Design review of the part built by this model. Coordinates are the model's own, in mm. Face numbers are marked on the shaded views. A direction names the side the tool comes from. Give positions to 0.01 mm unless a question says otherwise; leave off trailing zeros. Loops run counter-clockwise (first coordinate to the right, second up) from the corner with the lowest first, then second, coordinate; pieces in that order, holes last. Notation, with made-up numbers: (86, 47.5) -> (117, 47.5) arc R10 cw to (117, 57.5) -> close; hole circle Ø8 at (19.25, 5.25). An arc over 180 degrees is marked (long way). Answer in a Markdown table with one row per item. Add a question column.
(1) For line 1 (X direction, y = -5, z = 21.25); line 2 (Y direction, x = 7.75, z = 1), list the stretches that pass through material, from the lowest coordinate up.
(2) Consider section B-B on x = 4.5. Write out the cut boundary in (y, z).
(3) For the marked faces 1 and 2, list the 3-axis set-ups (+Z, -Z, +X, -X, +Y, -Y) from which the entire face can be reached by the end or side of a thin tool; tool diameter is ignored.
(4) Consider section D-D on x = 10. Write out the cut boundary in (y, z), then the cut area to 3 significant figures.
(5) Consider section A-A on z = 14. Write out the cut boundary in (x, y), then the cut area to 3 significant figures.
(6) Consider section C-C on z = 23. Write out the cut boundary in (x, y).
(7) For pin 1 (10 mm diameter, centred on x = 23.5, z = 11, fed in from +Y); pin 2 (7.5 mm diameter, centred on y = -48, z = 7, fed in from +X); pin 3 (8 mm diameter, centred on x = 13.5, y = -8.5, fed in from -Z) (1 decimal), all flat-tipped, find the tip position at first contact; note any pin that passes through.
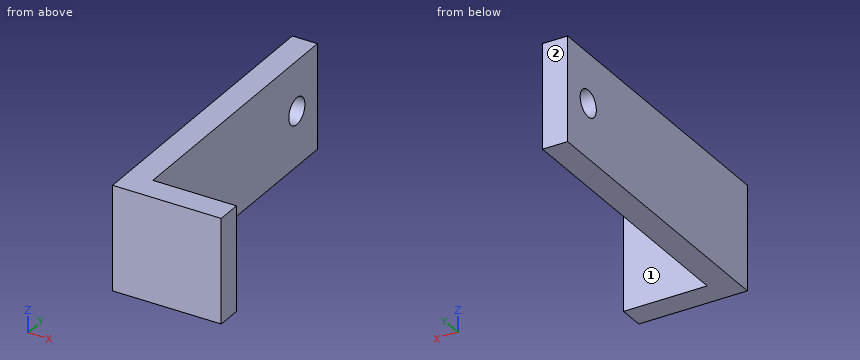
from build123d import *

# Parameters (mm, degrees)
SKETCH1_W           = 25
SKETCH1_H           = 71
BOSS_EXTRUDE1_DEPTH = 6
SKETCH2_W           = 25
SKETCH2_H           = 6
BOSS_EXTRUDE2_DEPTH = 20
SKETCH3_R           = 3.187620356
CUT_EXTRUDE1_DEPTH  = 22.5


with BuildPart() as part:
    # Sketch1 → Boss-Extrude1 (new body)
    with BuildSketch(Plane(origin=(0, 0, 0), x_dir=(0, 0, -1), z_dir=(1, 0, 0))):
        with Locations((-12.5, -35.5)):
            Rectangle(SKETCH1_W, SKETCH1_H)
    extrude(amount=BOSS_EXTRUDE1_DEPTH)

    # Sketch2 → Boss-Extrude2 (add)
    with BuildSketch(Plane(origin=(6, 0, 0), x_dir=(0, 0, -1), z_dir=(1, 0, 0))):
        with Locations((-12.5, -68)):
            Rectangle(SKETCH2_W, SKETCH2_H)
    extrude(amount=BOSS_EXTRUDE2_DEPTH)

    # Sketch3 → Cut-Extrude1 (cut)
    with BuildSketch(Plane(origin=(6, 0, 0), x_dir=(0, 0, -1), z_dir=(1, 0, 0))):
        with Locations((-13.070218864, -8.129494521)):
            Circle(SKETCH3_R)
    extrude(amount=-CUT_EXTRUDE1_DEPTH, mode=Mode.SUBTRACT)


solid = part.part
Values follow:
| question | item | result |
|---|---|---|
| 1 | line 1 | 0 to 6 |
| 1 | line 2 | -71 to -65 |
| 2 | outline | (-71, 0) -> (0, 0) -> (0, 25) -> (-71, 25) -> close; hole circle Ø6.38 at (-8.13, 13.07) |
| 3 | face 1 | +Z, -Z, +X, +Y |
| 3 | face 2 | +Z, -Z, +X, -X, +Y |
| 4 | outline | (-71, 0) -> (-65, 0) -> (-65, 25) -> (-71, 25) -> close |
| 4 | area | 150 mm2 |
| 5 | outline | (0, -71) -> (26, -71) -> (26, -65) -> (6, -65) -> (6, -11.18) -> (0, -11.18) -> close; (0, -5.08) -> (6, -5.08) -> (6, 0) -> (0, 0) -> close |
| 5 | area | 509 mm2 |
| 6 | outline | (0, -71) -> (26, -71) -> (26, -65) -> (6, -65) -> (6, 0) -> (0, 0) -> close |
| 7 | pin 1 | y = -65 |
| 7 | pin 2 | x = 6 |
| 7 | pin 3 | through |
